Autodesk Inventor part; units mm, degrees
ref_plane "YZ Plane" through (0, 0, 0) normal (1, 0, 0) x (0, 1, 0)
ref_plane "XZ Plane" through (0, 0, 0) normal (0, 1, 0) x (-1, 0, 0)
ref_plane "XY Plane" through (0, 0, 0) normal (0, 0, 1) x (1, 0, 0)
sketch "Sketch1" plane through (0, 0, 0) normal (1, 0, 0) x (0, 1, 0)
  line L0 (0, 0) -> (52, 0)
  line L1 (52, 0) -> (52, -53)
  line L2 (52, -53) -> (0, -53)
  line L3 (0, -53) -> (0, 0)
  line L4 (0, 0) -> (2.5, 0) construction
  line L5 (2.5, 0) -> (2.5, -2.5) construction
  line L6 (52, -53) -> (52, -50.5) construction
  line L7 (52, 0) -> (52, -2.5) construction
  line L8 (2.5, -2.5) -> (52, -2.5)
  line L9 (52, -2.5) -> (52, -50.5)
  line L10 (52, -50.5) -> (2.5, -50.5)
  line L11 (2.5, -50.5) -> (2.5, -2.5)
  dimension "d0" = 53
  dimension "d1" = 52
  dimension "d2" = 2.5
  dimension "d3" = 2.5
  dimension "d4" = 2.5
  dimension "d5" = 2.5
extrude "Extrusion1" add sketch "Sketch1" along normal blind 12.5 contours L0 L1 L8 L11 L10 L2 L3
sketch "Sketch2" plane through (0, 52, -50.5) normal (0, 1, 0) x (1, 0, 0)
  line L0 (12.5, 2.5) -> (12.5, 0) construction
  line L1 (12.5, 2.5) -> (11.5, 2.5) construction
  line L2 (0, 2.5) -> (12.5, 2.5) construction
  line L3 (11.5, 2.5) -> (11.5, 1.5) construction
  line L4 (0, 2.5) -> (1, 2.5) construction
  line L5 (1, 2.5) -> (1, 1.5) construction
  line L6 (0, -50.5) -> (12.5, -50.5) construction
  line L7 (12.5, -50.5) -> (11.5, -50.5) construction
  line L8 (11.5, -50.5) -> (11.5, -49.5) construction
  line L9 (0, -50.5) -> (1, -50.5) construction
  line L10 (1, -50.5) -> (1, -49.5) construction
  line L11 (1, -49.5) -> (11.5, -49.5)
  line L12 (11.5, -49.5) -> (11.5, -48)
  line L13 (11.5, -48) -> (1, -48)
  line L14 (1, -48) -> (1, -49.5)
  line L15 (1, 1.5) -> (11.5, 1.5)
  line L16 (11.5, 1.5) -> (11.5, 0)
  line L17 (11.5, 0) -> (1, 0)
  line L18 (1, 0) -> (1, 1.5)
  dimension "d8" = 1
  dimension "d9" = 1
  dimension "d10" = 1
  dimension "d11" = 1
  dimension "d14" = 1
  dimension "d15" = 1
  dimension "d16" = 1
  dimension "d17" = 1
  dimension "d18" = 1.5
  dimension "d19" = 10.5
  dimension "d20" = 10.5
  dimension "d21" = 1.5
extrude "Extrusion2" cut sketch "Sketch2" against normal blind 51
sketch "Sketch3" plane through (0, 2.5, -2.5) normal (0, 1, 0) x (1, 0, 0)
  line L0 (0, -2.5) -> (1, -2.5) construction
  line L1 (0, -2.5) -> (12.5, -2.5) construction
  line L2 (0, -2.5) -> (0, -1.5) construction
  line L3 (0, -2.5) -> (0, 50.5) construction
  line L4 (0, -1.5) -> (1, -1.5) construction
  line L5 (1, -1.5) -> (11.5, -1.5)
  line L6 (11.5, -1.5) -> (11.5, 49.5)
  line L7 (11.5, 49.5) -> (1, 49.5)
  line L8 (1, 49.5) -> (1, -1.5)
  dimension "d23" = 1
  dimension "d24" = 1
  dimension "d25" = 10.5
  dimension "d26" = 51
extrude "Extrusion3" cut sketch "Sketch3" against normal blind 1.5
sketch "Sketch4" plane through (12.5, 0, 0) normal (1, 0, 0) x (0, 0, -1)
  line L0 (53, 52) -> (50.5, 52) construction
  line L1 (53, 52) -> (53, 26.5) construction
  line L2 (53, 26.5) -> (108.8773, 26.5) construction
  line L3 (53, 26.5) -> (53, 31.5) construction
  line L4 (53, 0) -> (53, 52) construction
  line L5 (53, 31.5) -> (88, 31.5)
  line L6 (88, 31.5) -> (88, 21.5)
  line L7 (88, 21.5) -> (53, 21.5)
  line L8 (53, 21.5) -> (53, 31.5)
  line L9 (0, 52) -> (0, 26.5) construction
  line L10 (0, 52) -> (0, 0) construction
  line L11 (0, 26.5) -> (-54.8348, 26.5) construction
  line L12 (0, 26.5) -> (0, 31.5) construction
  line L13 (0, 31.5) -> (-35, 31.5)
  line L14 (-35, 31.5) -> (-35, 21.5)
  line L15 (-35, 21.5) -> (0, 21.5)
  line L16 (0, 21.5) -> (0, 31.5)
  dimension "d29" = 25.5
  dimension "d30" = 5
  dimension "d31" = 10
  dimension "d32" = 35
  dimension "d41" = 25.5
  dimension "d42" = 5
  dimension "d43" = 35
  dimension "d44" = 10
extrude "Extrusion4" add sketch "Sketch4" against normal blind 12.5
sketch "Sketch5" plane through (12.5, 0, 0) normal (1, 0, 0) x (0, 0, -1)
  line L0 (53, 52) -> (50.5, 52) construction
  line L1 (50.5, 52) -> (50.5, 26.5) construction
  line L2 (50.5, 52) -> (50.5, 2.5) construction
  line L3 (50.5, 26.5) -> (53, 26.5) construction
  line L4 (53, 26.5) -> (57, 26.5) construction
  circle A0 centre (57, 26.5) radius 3
  line L5 (57, 26.5) -> (82.2, 26.5) construction
  circle A1 centre (82.2, 26.5) radius 3
  line L6 (0, 52) -> (0, 26.5) construction
  line L7 (0, 26.5) -> (-4, 26.5) construction
  line L8 (-4, 26.5) -> (-29.2, 26.5) construction
  circle A2 centre (-4, 26.5) radius 3
  circle A3 centre (-29.2, 26.5) radius 3
  point P0 (0, 0)
  dimension "d35" = 25.5
  dimension "d36" = 2.5
  dimension "d37" = 6
  dimension "d38" = 4
  dimension "d39" = 25.2
  dimension "d40" = 6
  dimension "d45" = 25.5
  dimension "d46" = 4
  dimension "d47" = 25.2
  dimension "d48" = 6
  dimension "d49" = 6
extrude "Extrusion5" cut sketch "Sketch5" against normal blind 12.5
sketch "Sketch6" plane through (0, 0, -53) normal (0, -1, 0) x (1, 0, 0)
  line L0 (12.5, 53) -> (0, 53)
  line L1 (0, 53) -> (0, 0)
  line L2 (0, 0) -> (12.5, 0)
  line L3 (12.5, 0) -> (12.5, 53)
  line L4 (12.5, 53) -> (12.5, 0)
  dimension "d54" = 0
extrude "Extrusion6" add sketch "Sketch6" along normal blind 4
sketch "Sketch7" plane through (0, -4, -53) normal (0, -1, 0) x (1, 0, 0)
  line L0 (12.5, 53) -> (0, 53) construction
  line L1 (6.25, 53) -> (6.25, 26.5) construction
  circle A0 centre (6.25, 26.5) radius 0.5
  dimension "d55" = 26.5
  dimension "d56" = 1
extrude "Extrusion7" cut sketch "Sketch7" against normal blind 1
equation "\"d0\" = lfan + 2 * thickness"
equation "\"d1\" = lfan + thickness"
equation "\"d2\" = fanclip"
equation "\"d3\" = fanclip"
equation "\"d4\" = fanclip"
equation "\"d5\" = fanclip"
equation "\"d6\" = tfan + 2 * thickness"
equation "\"d8\" = thickness"
equation "\"d9\" = thickness"
equation "\"d10\" = thickness"
equation "\"d11\" = thickness"
equation "\"d14\" = thickness"
equation "\"d15\" = thickness"
equation "\"d16\" = thickness"
equation "\"d17\" = thickness"
equation "\"d18\" = fanclip - thickness"
equation "\"d19\" = tfan"
equation "\"d20\" = tfan"
equation "\"d21\" = fanclip - thickness"
equation "\"d12\" = lfan"
equation "\"d23\" = thickness"
equation "\"d24\" = thickness"
equation "\"d25\" = tfan"
equation "\"d26\" = lfan"
equation "\"d27\" = fanclip - thickness"
equation "\"d29\" = 0.5 * lfan"
equation "\"d30\" = 0.5 * twing"
equation "\"d31\" = twing"
equation "\"d32\" = lwing"
equation "\"d41\" = 0.5 * lfan"
equation "\"d42\" = 0.5 * twing"
equation "\"d43\" = lwing"
equation "\"d44\" = twing"
equation "\"d33\" = tfan + 2 * thickness"
equation "\"d35\" = 0.5 * lfan"
equation "\"d36\" = fanclip"
equation "\"d37\" = dPhoto"
equation "\"d38\" = gapto1"
equation "\"d39\" = gapto2"
equation "\"d40\" = dPhoto"
equation "\"d45\" = 0.5 * lfan"
equation "\"d46\" = gapto1"
equation "\"d47\" = gapto2"
equation "\"d48\" = dPhoto"
equation "\"d49\" = dPhoto"
equation "\"d50\" = tfan + 2 * thickness"
equation "\"d52\" = 4 * thickness"
equation "\"d55\" = 0.5 * lfan + thickness"
equation "\"d57\" = thickness"
equation "\"lfan\" = 51"
equation "\"tfan\" = 10.5"
equation "\"thickness\" = 1"
equation "\"fanclip\" = 2.5"
equation "\"twing\" = 10"
equation "\"lwing\" = 35"
equation "\"dPhoto\" = 6"
equation "\"gapto1\" = 4"
equation "\"gapto2\" = 25.2"
properties part number "FanPTMounts"
Check sheet for the modelled part. Datum: model origin and axes. Units: mm. A direction names the side the tool comes from. Give positions to 0.01 mm unless a question says otherwise; leave off trailing zeros. Write each loop counter-clockwise with the first axis right and the second up, starting at its lowest first coordinate (ties: lowest second). Pieces come first, ordered by that corner, then holes. Notation, with made-up numbers: (54.25, 82.25) -> (106.25, 82.25) arc R4 ccw to (106.25, 87.25) -> close; hole circle Ø3 at (62.25, 29.25). An arc over 180 degrees is marked (long way). Use CSV: the item, a comma, the result in double quotes. Start each with the question number.
Q1. Release check for a two-part mould opening along Z. For faces 5 (the flat face through (1, 2, -27)), 6 (the flat face through (6, 27, 35)), 7 (the flat face through (12.5, 1, -27)), 8 (the cylindrical face through (6.3, 24.7, -79.8)) record: +Z half, -Z half, draft (parallel to the pull), parting line (faces both ways), or undercut.
Q2. Cross-section at C-C on x = 9. Enter the section's corners in (y, z), and give its area (3 significant figures).
Q3. Scan lines: line 1 along Y through (x, z) = (8.5, -82); line 2 along Z through (x, y) = (4.25, 22); line 3 along Z through (x, y) = (4.75, 12). Record each from-to range of solid material in increasing order.
Q4. Tool access check on faces 1 (the flat face through (6, 31.5, -70)), 2 (the flat face through (6, 27, -52)), 3 (the flat face through (6, 9, -53)), 4 (the flat face through (6, 21.5, 18)). Record the directions out of +Z, -Z, +X, -X, +Y, -Y that give a thin tool (end or side, any length) a straight path to the whole face; none if there is none.
Q5. Cross-section at D-D on z = -12. Enter the section's corners in (x, y), and give its area (3 significant figures).
Q6. Depth check by flat-ended pin: P1, Ø6, axis at x = 5, z = 18.5, coming from the +Y side; P2, Ø3, axis at x = 7.5, y = 14.5, coming from the -Z side; P3, Ø4, axis at x = 5.5, y = 45, coming from the +Z side. Enter the tip coordinate at first touch or a pass-through.
Q7. Cross-section at A-A on y = 9. Enter the section's corners in (x, z).
Q8. Cross-section at B-B on z = 29.2. Enter the section's corners in (x, y), and give its area (3 significant figures).
Working result:
1,face 5,"undercut"
1,face 6,"+Z half"
1,face 7,"draft"
1,face 8,"undercut"
2,outline,"(-4, -53) -> (21.5, -53) -> (21.5, -88) -> (31.5, -88) -> (31.5, -53) -> (52, -53) -> (52, -52) -> (1, -52) -> (1, -1) -> (52, -1) -> (52, 0) -> (31.5, 0) -> (31.5, 35) -> (21.5, 35) -> (21.5, 0) -> (-4, 0) -> close; hole circle Ø6 at (26.5, -82.2); hole circle Ø6 at (26.5, -57); hole circle Ø6 at (26.5, 4); hole circle Ø6 at (26.5, 29.2)"
2,area,"954 mm^2"
3,line 1,"y = 21.5 to 23.51, 29.49 to 31.5"
3,line 2,"z = -88 to -52, -1 to 35"
3,line 3,"z = -53 to -52, -1 to 0"
4,face 1,"-Z, +X, -X, +Y"
4,face 2,"+Y"
4,face 3,"-Z, +X, -X, -Y"
4,face 4,"+Z, +X, -X, -Y"
5,outline,"(0, -4) -> (12.5, -4) -> (12.5, 2.5) -> (11.5, 2.5) -> (11.5, 1) -> (1, 1) -> (1, 2.5) -> (0, 2.5) -> close"
5,area,"65.5 mm^2"
6,P1,"stops at y = 31.5"
6,P2,"stops at z = -53"
6,P3,"stops at z = 0"
7,outline,"(0, -53) -> (12.5, -53) -> (12.5, -50.5) -> (11.5, -50.5) -> (11.5, -52) -> (1, -52) -> (1, -50.5) -> (0, -50.5) -> close; (0, -2.5) -> (1, -2.5) -> (1, -1) -> (11.5, -1) -> (11.5, -2.5) -> (12.5, -2.5) -> (12.5, 0) -> (0, 0) -> close"
8,outline,"(0, 21.5) -> (12.5, 21.5) -> (12.5, 23.5) -> (0, 23.5) -> close; (0, 29.5) -> (12.5, 29.5) -> (12.5, 31.5) -> (0, 31.5) -> close"
8,area,"50.0 mm^2"
